Geometry check sheet. Reference: drawing and pictorial views, mm from the part's lowest x, y, z. A direction names the side the tool comes from. Coordinates: 2 decimals unless noted, no trailing zeros. Write each loop counter-clockwise with the first axis right and the second up, starting at its lowest first coordinate (ties: lowest second). Pieces come first, ordered by that corner, then holes. Notation, with made-up numbers: (14, 19) -> (30, 19) arc R28 cw to (30, 43) -> close; hole circle Ø5 at (41, 50). An arc over 180 degrees is marked (long way). Use a Markdown table: item, result.
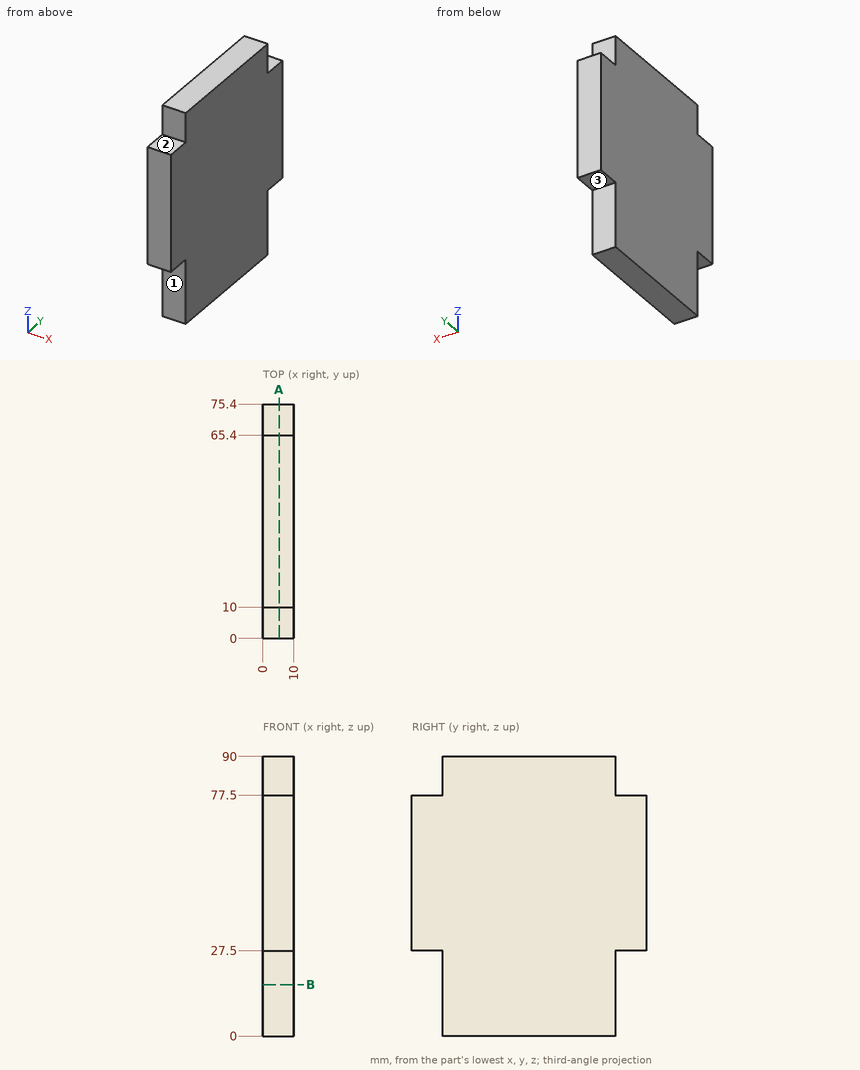
Item 1: Thickness scan on L1, parallel to Y at x = 5.5, z = 21; L2, parallel to Z at x = 4.75, y = 70. Record the ranges inside material, lowest first. Write a range as [from, to].
Answer block:
| item | result |
|---|---|
| L1 | y = [10, 65.4] |
| L2 | z = [27.5, 77.5] |
Item 2: Depth check by flat-ended pin: P1, Ø3, axis at x = 9, y = 28.5, coming from the -Z side; P2, Ø3, axis at x = 4, y = 4.5, coming from the +Z side; P3, Ø3, axis at x = 7, z = 81, coming from the -Y side; P4, Ø3, axis at x = 3, z = 8.5, coming from the +Y side. Enter the tip coordinate at first touch or a pass-through.
Answer block:
| item | result |
|---|---|
| P1 | stops at z = 0 |
| P2 | stops at z = 77.5 |
| P3 | stops at y = 10 |
| P4 | stops at y = 65.4 |
Item 3: Section check A-A on x = 5.25. Record the boundary of the cut face in (y, z).
Answer block:
| item | result |
|---|---|
| outline | (0, 27.5) -> (10, 27.5) -> (10, 0) -> (65.4, 0) -> (65.4, 27.5) -> (75.4, 27.5) -> (75.4, 77.5) -> (65.4, 77.5) -> (65.4, 90) -> (10, 90) -> (10, 77.5) -> (0, 77.5) -> close |
Item 4: Tool access check on the marked faces 1, 2 and 3. Record the directions out of +Z, -Z, +X, -X, +Y, -Y that give a thin tool (end or side, any length) a straight path to the whole face; none if there is none.
Answer block:
| item | result |
|---|---|
| face 1 | -Z, +X, -X, -Y |
| face 2 | +Z, +X, -X, -Y |
| face 3 | -Z, +X, -X, +Y |
Item 5: Section check B-B on z = 16.5. Record the boundary of the cut face in (x, y), then the cut area to 3 significant figures.
Answer block:
| item | result |
|---|---|
| outline | (0, 10) -> (10, 10) -> (10, 65.4) -> (0, 65.4) -> close |
| area | 554 mm^2 |
